from build123d import *

# Parameters (mm, degrees)
F0_R     = 3.5
F0_W     = 30
F0_H     = 2.5
F1_DEPTH = 2.5
F2_DEPTH = 12.5
F3_DEPTH = 32.5
F4_R     = 1.75
F5_DEPTH = 2.501


with BuildPart() as f1:
    # F0 (on Top) → F1 (new body)
    with BuildSketch(Plane.XY):
        Polygon((-15, 13.75), (-15, -16.25), (6.69e-08, -16.25), (15, -16.25), (15, 13.75), align=None)
        with BuildLine():
            ThreePointArc((6, -10.25), (4.2426407108, -14.4926406635), (6.69e-08, -16.25))
            ThreePointArc((6.69e-08, -16.25), (-4.2426407108, -6.0073593365), (6, -10.25))
        make_face(mode=Mode.SUBTRACT)
        with BuildLine():
            ThreePointArc((6, -10.25), (-4.2426407108, -6.0073593365), (6.69e-08, -16.25))
            ThreePointArc((6.69e-08, -16.25), (4.2426407108, -14.4926406635), (6, -10.25))
        make_face()
        with Locations((0, -10.25)):
            Circle(F0_R, mode=Mode.SUBTRACT)
        with Locations((0, 15)):
            Rectangle(F0_W, F0_H)
        with Locations((0, -10.25)):
            Circle(F0_R)
    extrude(amount=F1_DEPTH)

    # F0 (on Top) → F2 (join)
    with BuildSketch(Plane.XY):
        with BuildLine():
            ThreePointArc((6, -10.25), (-4.2426407108, -6.0073593365), (6.69e-08, -16.25))
            ThreePointArc((6.69e-08, -16.25), (4.2426407108, -14.4926406635), (6, -10.25))
        make_face()
        with Locations((0, -10.25)):
            Circle(F0_R, mode=Mode.SUBTRACT)
    extrude(amount=F2_DEPTH)

    # F0 (on Top) → F3 (join)
    with BuildSketch(Plane.XY):
        with Locations((0, 15)):
            Rectangle(F0_W, F0_H)
    extrude(amount=F3_DEPTH)

    # F4 (on face) → F5 (cut, through all)
    with BuildSketch(Plane.XZ.offset(-13.75)):
        with Locations((0, 25)):
            Circle(F4_R)
    extrude(amount=-F5_DEPTH, mode=Mode.SUBTRACT)


solid = f1.part
The listing builds one solid part. Answer for the finished solid, in the listing's coordinates (mm). A direction names the side the tool comes from. Give positions to 0.01 mm unless a question says otherwise; leave off trailing zeros. Loops run counter-clockwise (first coordinate to the right, second up) from the corner with the lowest first, then second, coordinate; pieces in that order, holes last. Notation, with made-up numbers: (-5, -21.75) - (23, -21.75) arc R31 ccw to (23, 6.25) - close; hole circle Ø1 at (-5.5, 35.25). An arc over 180 degrees is marked (long way). Answer as a JSON object with one key per item and string values.
1. For faces 1 (the cylindrical face through (-0.759, -13.667, 7.43)), 2 (the flat face through (3, -13, 12.5)), 3 (the flat face through (0, 15, 32.5)), determine the directions among +Z, -Z, +X, -X, +Y, -Y from which every point of the face is accessible in a straight line to the end or side of a thin tool.
Determined:
{"face 1": "+Z", "face 2": "+Z, +X, -X, -Y", "face 3": "+Z, +X, -X, +Y, -Y"}
2. A cutting plane is placed at B-B (x = -8.75). Write down the section's boundary in (y, z).
Determined:
{"outline": "(-16.25, 0) - (16.25, 0) - (16.25, 32.5) - (13.75, 32.5) - (13.75, 2.5) - (-16.25, 2.5) - close"}
3. For a pull along Y with two mould halves and no side action, classify faces 4 (the cylindrical face through (-0.228, 14.982, 26.735)), 5 (the flat face through (0, -10, 2.5)), 6 (the flat face through (0, -16.25, 1)), 7 (the flat face through (0, -1, 2.5)) as pulls with the +Y half, pulls with the -Y half, needs draft (parallel to the pull), parting line crosses it, or undercut.
Determined:
{"face 4": "needs draft", "face 5": "undercut", "face 6": "pulls with the -Y half", "face 7": "undercut"}
4. A cutting plane is placed at C-C (y = -11). Write down the section's boundary in (x, z).
Determined:
{"outline": "(-15, 0) - (15, 0) - (15, 2.5) - (5.95, 2.5) - (5.95, 12.5) - (3.42, 12.5) - (3.42, 2.5) - (-3.42, 2.5) - (-3.42, 12.5) - (-5.95, 12.5) - (-5.95, 2.5) - (-15, 2.5) - close"}
5. A cutting plane is placed at A-A (z = 25). Write down the section's boundary in (x, y), then the cut area to 4 significant figures.
Determined:
{"outline": "(-15, 13.75) - (-1.75, 13.75) - (-1.75, 16.25) - (-15, 16.25) - close; (1.75, 13.75) - (15, 13.75) - (15, 16.25) - (1.75, 16.25) - close", "area": "66.25 mm²"}
6. Find the intervals of material crossed by L1, parallel to X at y = -10.25, z = 4.5; L2, parallel to Z at x = 0, y = 15.2; L3, parallel to Y at x = -1.5, z = 8, in increasing order. Write a range as [from, to].
Determined:
{"L1": "[-6, -3.5], [3.5, 6]", "L2": "[0, 23.25], [26.75, 32.5]", "L3": "[-16.06, -13.41], [-7.09, -4.44], [13.75, 16.25]"}
7. Flat-ended cylindrical pins translate along their axes: pin 1 Ø8 at (x, y) = (0, -10.25) entering from +Z; pin 2 Ø5 at (x, z) = (-7.5, 21.5) entering from -Y; pin 3 Ø9 at (x, y) = (2, 2.5) entering from +Z; pin 4 Ø2 at (x, z) = (0, 25) entering from +Y. Find the tip coordinate at first contact, or state that the pin passes through.
Determined:
{"pin 1": "z = 12.5", "pin 2": "y = 13.75", "pin 3": "z = 2.5", "pin 4": "through"}
8. A cutting plane is placed at D-D (z = 13.5). Write down the section's boundary in (x, y), then the cut area to 3 significant figures.
Determined:
{"outline": "(-15, 13.75) - (15, 13.75) - (15, 16.25) - (-15, 16.25) - close", "area": "75.0 mm²"}
